from build123d import *

# Parameters (mm, degrees)
F0_W      = 15.875
F0_H      = 7.9375
F0_R      = 2.38125
F1_DEPTH  = 3.175
F2_DEPTH  = 4.7625
F3_T      = -1.5875
F4_R      = 1.5875
F4_R_2    = 0.79375
F5_DEPTH  = 1.5875
F6_W      = 1.5875
F6_H      = 6.35
F7_DEPTH  = 4.7625
F8_W      = 1.5875
F8_H      = 0.79375
F9_DEPTH  = 3.175
F10_DEPTH = 25.4


with BuildPart() as f1:
    # F0 (on Top) → F1 (new body)
    with BuildSketch(Plane.XY):
        Rectangle(F0_W, F0_H)
        with Locations((-3.96875, 0)):
            Circle(F0_R, mode=Mode.SUBTRACT)
        with Locations((3.96875, 0)):
            Circle(F0_R, mode=Mode.SUBTRACT)
    extrude(amount=F1_DEPTH)

    # F0 (on Top) → F2 (join)
    with BuildSketch(Plane.XY):
        with Locations((3.96875, 0)):
            Circle(F0_R)
        with Locations((-3.96875, 0)):
            Circle(F0_R)
    extrude(amount=F2_DEPTH)

    # F3
    f3_openings = [f1.faces().sort_by_distance(p)[0] for p in [
        (0, 0, 0),
    ]]
    offset(amount=F3_T, openings=f3_openings, kind=Kind.INTERSECTION)

    # F4 (on face) → F5 (join)
    with BuildSketch(Plane(origin=(0, 0, 1.5875), x_dir=(1, 0, 0), z_dir=(0, 0, -1))):
        Circle(F4_R)
        Circle(F4_R_2, mode=Mode.SUBTRACT)
    extrude(amount=F5_DEPTH)

    # F6 (on face) → F7 (join)
    with BuildSketch(Plane.YZ.offset(7.9375)):
        with Locations((0.79375, 3.175)):
            Rectangle(F6_W, F6_H)
        with Locations((-0.79375, 3.175)):
            Rectangle(F6_W, F6_H)
    extrude(amount=F7_DEPTH)

    # F8 (on face) → F9 (join)
    with BuildSketch(Plane.XZ.offset(1.5875)):
        with BuildLine():
            Line((12.7, 0), (10.5999348968, 0))
            ThreePointArc((10.5999348968, 0), (11.5774679849, -0.5886905508), (12.7, -0.79375))
            Line((12.7, -0.79375), (12.7, 0))
        make_face()
        with BuildLine():
            Line((12.7, 0), (12.7, -0.79375))
            ThreePointArc((12.7, -0.79375), (13.5217504682, -0.6855644985), (14.2875, -0.368380657))
            Line((14.2875, -0.368380657), (14.2875, 0))
            Line((14.2875, 0), (12.7, 0))
        make_face()
        with BuildLine():
            ThreePointArc((14.2875, 5.130880657), (13.5217504682, 5.4480644985), (12.7, 5.55625))
            Line((12.7, 5.55625), (12.7, 3.96875))
            Line((12.7, 3.96875), (14.2875, 3.96875))
            Line((14.2875, 3.96875), (14.2875, 5.130880657))
        make_face()
        with Locations((13.49375, 0.396875)):
            Rectangle(F8_W, F8_H)
    extrude(amount=-F9_DEPTH)

    # F8 (on face) → F10 (cut)
    with BuildSketch(Plane.XZ.offset(1.5875)):
        with BuildLine():
            Line((7.9375, 6.35), (7.9375, 3.175))
            Line((7.9375, 3.175), (7.9375, 2.38125))
            Line((7.9375, 2.38125), (9.525, 2.38125))
            ThreePointArc((9.525, 2.38125), (10.4549359697, 4.6263140303), (12.7, 5.55625))
            Line((12.7, 5.55625), (12.7, 6.35))
            Line((12.7, 6.35), (7.9375, 6.35))
        make_face()
        with BuildLine():
            Line((12.7, 2.38125), (11.1125, 2.38125))
            ThreePointArc((11.1125, 2.38125), (11.5774679849, 1.2587179849), (12.7, 0.79375))
            Line((12.7, 0.79375), (12.7, 2.38125))
        make_face()
        with BuildLine():
            ThreePointArc((12.7, 3.96875), (11.5774679849, 3.5037820151), (11.1125, 2.38125))
            Line((11.1125, 2.38125), (12.7, 2.38125))
            Line((12.7, 2.38125), (12.7, 3.96875))
        make_face()
    extrude(amount=-F10_DEPTH, mode=Mode.SUBTRACT)


solid = f1.part
Verification items for the finished model (mm, model axes). A direction names the side the tool comes from. Coordinates: 2 decimals unless noted, no trailing zeros. Write each loop counter-clockwise with the first axis right and the second up, starting at its lowest first coordinate (ties: lowest second). Pieces come first, ordered by that corner, then holes. Notation, with made-up numbers: M 9.25,43.5 L 53.25,43.5 A13 ccw 53.25,66.5 Z; hole C 59,57 d8. An arc over 180 degrees is marked long. Use a Markdown table: item, result.
Q1. Thickness scan on line 1 (Y direction, x = 0, z = 0.45); line 2 (X direction, y = 0, z = 0.4); line 3 (X direction, y = 0, z = 2.35) (1 decimal). Record the ranges inside material, lowest first.
Reply:
| item | result |
|---|---|
| line 1 | y = -3.97 to -2.38, -1.59 to -0.79, 0.79 to 1.59, 2.38 to 3.97 |
| line 2 | x = -7.94 to -6.35, -1.59 to -0.79, 0.79 to 1.59, 6.35 to 14.29 |
| line 3 | x = -7.9 to -4.8, -3.2 to 3.2, 4.8 to 11.1 |
Q2. Sectioned sample at B-B, the plane z = 2.75. Record the boundary of the cut face in (x, y) (1 decimal), plus the area to 3 significant figures.
Reply:
| item | result |
|---|---|
| outline | M -7.9,-4 L 7.9,-4 L 7.9,4 L -7.9,4 Z; M 9.5,-1.6 L 11.2,-1.6 L 11.2,1.6 L 9.5,1.6 Z; hole C -4,0 d1.6; hole C 4,0 d1.6 |
| area | 127 mm² |
Q3. Set-up check for faces 4 (the face through (1, -3, 0)), 5 (the face through (6.24, 0.72, 3.96)), 6 (the face through (-4, 0, 4.762)), 7 (the face through (13, 0, 3.969)), 8 (the face through (0, -2.381, 1)): record each of +Z, -Z, +X, -X, +Y, -Y from which the full face is reachable in a straight line by a thin tool's end or side.
Reply:
| item | result |
|---|---|
| face 4 | -Z, -X, +Y, -Y |
| face 5 | +Z |
| face 6 | +Z, -X, +Y, -Y |
| face 7 | +X, +Y, -Y |
| face 8 | -Z |
Q4. Go/stop test with flat-tipped pins: P1, Ø0.8, axis at x = 13.5, y = 0.5, coming from the -Z side; P2, Ø0.5, axis at x = 8.5, y = -0.5, coming from the +Z side; P3, Ø1, axis at x = 4, y = -2, coming from the +Z side; P4, Ø1, axis at y = 1.5, z = 3.5, coming from the +X side. Record where each tip stops, or that it passes through.
Reply:
| item | result |
|---|---|
| P1 | stops at z = -0.77 |
| P2 | stops at z = 2.38 |
| P3 | stops at z = 4.76 |
| P4 | stops at x = 14.29 |
Q5. Sectioned sample at A-A, the plane x = 0. Record the boundary of the cut face in (y, z) (1 decimal).
Reply:
| item | result |
|---|---|
| outline | M -4,0 L -2.4,0 L -2.4,1.6 L -1.6,1.6 L -1.6,0 L -0.8,0 L -0.8,1.6 L 0.8,1.6 L 0.8,0 L 1.6,0 L 1.6,1.6 L 2.4,1.6 L 2.4,0 L 4,0 L 4,3.2 L -4,3.2 Z |
Q6. Sectioned sample at D-D, the plane z = 3.75. Record the boundary of the cut face in (x, y).
Reply:
| item | result |
|---|---|
| outline | C -3.97,0 d4.76; C 3.97,0 d4.76; M 9.84,-1.59 L 11.9,-1.59 L 11.9,1.59 L 9.84,1.59 Z |
Q7. Draft check along Y on faces 1 (the face through (0, 0, 1.588)), 2 (the face through (14.288, 0, 4.5)), 3 (the face through (11, 1.588, 2)). Enter one of: +Y half, -Y half, draft (parallel to the pull), parting line (faces both ways), or undercut.
Reply:
| item | result |
|---|---|
| face 1 | undercut |
| face 2 | draft |
| face 3 | +Y half |
